Could you check a few things on this model? Use its own coordinates, in mm. Face numbers are marked on the shaded views. A direction names the side the tool comes from. Give positions to 0.01 mm unless a question says otherwise; leave off trailing zeros. Loops run counter-clockwise (first coordinate to the right, second up) from the corner with the lowest first, then second, coordinate; pieces in that order, holes last. Notation, with made-up numbers: (-30, 46.5) -> (-21, 46.5) arc R11 ccw to (-21, 66.5) -> close; hole circle Ø3 at (-31, 82). An arc over 180 degrees is marked (long way). Write item = value, one per line. Start each with the question number.
1) I want a section at B-B (y = 6.5). List the corners of the cut face in (x, z) for me (3 decimals).
2) On a 3-axis mill with a long thin cutter (end or side, diameter ignored), from which of +Z, -Z, +X, -X, +Y, -Y can I reach the whole of each face in a straight line? I mean the marked faces 1 and 2. Say none if no direction works.
3) I'm going to push flat-ended pins straight in: pin 1 Ø2 at (x, y) = (3.5, 7.5) entering from +Z; pin 2 Ø7 at (y, z) = (11, -6.5) entering from +X; pin 3 Ø3 at (y, z) = (11, 14) entering from -X. Where does each tip first touch, or does it pass through?
4) I want a section at C-C (z = -1.5). List the corners of the cut face in (x, y) for me, and give its area (3 significant figures).
5) I want a section at A-A (x = 12.5). List the corners of the cut face in (y, z) for me.
6) I want a section at D-D (z = 4.5). List the corners of the cut face in (x, y) for me, and give its area (3 significant figures).
7) I need wall thicknesses on probe 1 along Y at (x, z) = (12.5, -2); probe 2 along X at (y, z) = (1, 15.5); probe 3 along Z at (x, y) = (2, 10.5). Which ranges of each line are inside material? Lowest first, please. Write a range as from..to.
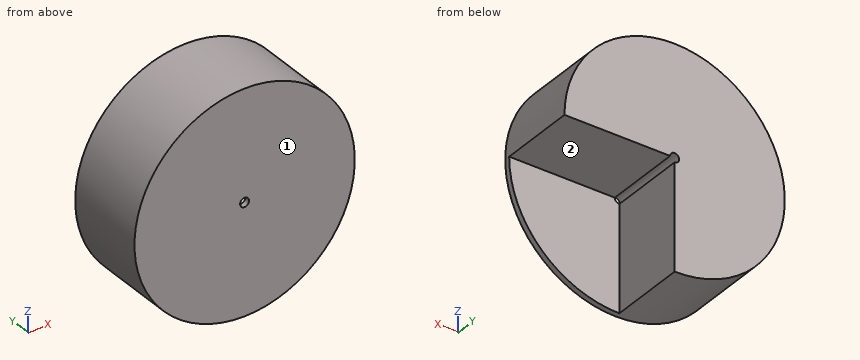
from build123d import *

# Parameters (mm, degrees)
SKETCH5_R           = 20
BOSS_EXTRUDE2_DEPTH = 15
CUT_EXTRUDE1_START  = -14
CUT_EXTRUDE1_DEPTH  = 14
SKETCH7_R           = 0.815
CUT_EXTRUDE2_DEPTH  = 150


with BuildPart() as part:
    # Sketch5 → Boss-Extrude2 (new body)
    with BuildSketch(Plane(origin=(0, 0, 0), x_dir=(1, 0, 0), z_dir=(0, 1, 0))):
        with Locations(Location((0, 0, 0), (0, 0, 270))):
            Circle(SKETCH5_R)
    extrude(amount=BOSS_EXTRUDE2_DEPTH)

    # Sketch6 → Cut-Extrude1 (cut)
    with BuildSketch(Plane(origin=(0, 15, 0), x_dir=(1, 0, 0), z_dir=(0, 1, 0)).offset(CUT_EXTRUDE1_START)):
        with BuildLine():
            Line((0, 20), (0, 0))
            Line((0, 0), (20, 0))
            ThreePointArc((20, 0), (14.142135624, 14.142135624), (0, 20))
        make_face()
    extrude(amount=CUT_EXTRUDE1_DEPTH, mode=Mode.SUBTRACT)

    # Sketch7 → Cut-Extrude2 (cut)
    with BuildSketch(Plane(origin=(0, 15, 0), x_dir=(1, 0, 0), z_dir=(0, 1, 0))):
        with Locations(Location((0, 0, 0), (0, 0, 270))):
            Circle(SKETCH7_R)
    extrude(amount=-CUT_EXTRUDE2_DEPTH, mode=Mode.SUBTRACT)


solid = part.part
Answer list:
q1.outline = (0, -20) -> (0, -0.815) arc R0.815 cw (long way) to (0.815, 0) -> (20, 0) arc R20 ccw (long way) to start
q2.face_1 = +Z, -Z, +X, -X, -Y
q2.face_2 = -Z, +X, +Y
q3.pin_1 = 19.84
q3.pin_2 = 0
q3.pin_3 = -15.61
q4.outline = (-19.94, 0) -> (19.94, 0) -> (19.94, 1) -> (0, 1) -> (0, 15) -> (-19.94, 15) -> close
q4.area = 319 mm^2
q5.outline = (0, -15.61) -> (1, -15.61) -> (1, 0) -> (15, 0) -> (15, 15.61) -> (0, 15.61) -> close
q6.outline = (-19.49, 0) -> (19.49, 0) -> (19.49, 15) -> (-19.49, 15) -> close
q6.area = 585 mm^2
q7.probe_1 = 0..1
q7.probe_2 = -12.64..12.64
q7.probe_3 = 0..19.9
